Part model, mm, in its own coordinate system. Round coordinates to 2 decimals unless told otherwise and drop trailing zeros. Loops run counter-clockwise (first coordinate to the right, second up) from the corner with the lowest first, then second, coordinate; pieces in that order, holes last. Notation, with made-up numbers: (45.5, 17) -> (91.5, 17) arc R31 cw to (91.5, 54) -> close; hole circle Ø11 at (26.5, 68.25). An arc over 180 degrees is marked (long way). Answer as a JSON object with one key per item and string values. Group by question number.
from build123d import *

# Parameters (mm, degrees)
F0_W     = 1098.55
F0_H     = 317.5
F1_DEPTH = 3.175
F2_W     = 107.95
F2_H     = 82.55
F3_DEPTH = 38.1
F4_DEPTH = 1.5875
F5_W     = 101.6
F5_H     = 76.2
F6_DEPTH = 38.1


with BuildPart() as f1:
    # F0 (on Front) → F1 (new body)
    with BuildSketch(Plane.XZ):
        Rectangle(F0_W, F0_H)
    extrude(amount=F1_DEPTH)

    # F2 (on face) → F3 (join)
    with BuildSketch(Plane.XZ.offset(3.175)):
        with Locations((0, 92.075)):
            Rectangle(F2_W, F2_H)
    extrude(amount=-F3_DEPTH)

    # F2 (on face) → F4 (join)
    with BuildSketch(Plane.XZ.offset(3.175)):
        with Locations((0, 92.075)):
            Rectangle(F2_W, F2_H)
    extrude(amount=F4_DEPTH)

    # F5 (on face) → F6 (cut)
    with BuildSketch(Plane.XZ.offset(4.7625)):
        with Locations((0, 92.075)):
            Rectangle(F5_W, F5_H)
    extrude(amount=-F6_DEPTH, mode=Mode.SUBTRACT)


solid = f1.part
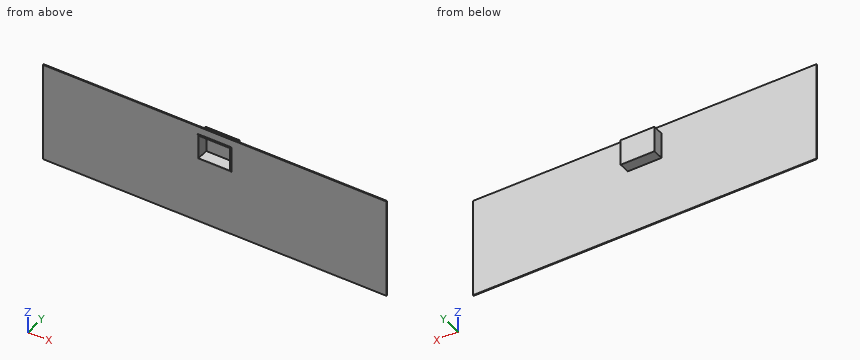
Item 1: Drill centre lines: line 1 (X direction, y = 6, z = 94) (3 decimals); line 2 (Y direction, x = 20.5, z = -78.5) (3 decimals); line 3 (Z direction, x = -22.5, y = 33) (3 decimals). Where is each one in solid material? Low to high.
Item 2: Drop flat-ended pins along their axis: pin 1 Ø10.5 at (x, y) = (-1, 16) entering from -Z; pin 2 Ø11.5 at (y, z) = (20.5, 105.5) entering from +X (3 decimals); pin 3 Ø19 at (y, z) = (12.5, 81) entering from -X (3 decimals); pin 4 Ø12 at (x, y) = (-386.5, 10.5) entering from +Z. Give the stop position or say it passes through.
Item 3: Band-saw the part on D-D, the plane z = -46. List the corners of the cut face in (x, y) (3 decimals), plus the area to 3 significant figures.
Item 4: Band-saw the part on B-B, the plane z = 95.5. List the corners of the cut face in (x, y) (1 decimal).
Item 5: Band-saw the part on A-A, the plane y = 22. List the corners of the cut face in (x, z) (3 decimals).
Item 6: Band-saw the part on C-C, the plane x = -218. List the corners of the cut face in (y, z) (3 decimals).
Entries:
{
 "1": {"line 1": "-53.975 to -50.8, 50.8 to 53.975", "line 2": "-3.175 to 0", "line 3": "50.8 to 53.975, 130.175 to 133.35"},
 "2": {"pin 1": "z = 50.8", "pin 2": "x = 53.975", "pin 3": "x = -53.975", "pin 4": "through"},
 "3": {"outline": "(-549.275, -3.175) -> (549.275, -3.175) -> (549.275, 0) -> (-549.275, 0) -> close", "area": "3,490 mm²"},
 "4": {"outline": "(-549.3, -3.2) -> (-54, -3.2) -> (-54, -4.8) -> (-50.8, -4.8) -> (-50.8, 33.3) -> (50.8, 33.3) -> (50.8, -4.8) -> (54, -4.8) -> (54, -3.2) -> (549.3, -3.2) -> (549.3, 0) -> (54, 0) -> (54, 34.9) -> (-54, 34.9) -> (-54, 0) -> (-549.3, 0) -> close"},
 "5": {"outline": "(-53.975, 50.8) -> (53.975, 50.8) -> (53.975, 133.35) -> (-53.975, 133.35) -> close; hole (-50.8, 53.975) -> (50.8, 53.975) -> (50.8, 130.175) -> (-50.8, 130.175) -> close"},
 "6": {"outline": "(-3.175, -158.75) -> (0, -158.75) -> (0, 158.75) -> (-3.175, 158.75) -> close"}
}
